from build123d import *

# Parameters (mm, degrees)
SKETCH1_W            = 34.3
SKETCH1_H            = 23.85
SKETCH1_W_2          = 24.3
SKETCH1_H_2          = 13.85
BOSS_EXTRUDE1_DEPTH  = 2
SKETCH4_W            = 8
SKETCH4_H            = 5
BOSS_EXTRUDE2_DEPTH  = 2
M2_CLEARANCE_HOLE1_D = 2.4
FILLET1_R            = 1
CUT_EXTRUDE1_DEPTH   = 3
FILLET2_R            = 0.25


with BuildPart() as part:
    # Sketch1 → Boss-Extrude1 (new body)
    with BuildSketch(Plane(origin=(0, 0, 0), x_dir=(1, 0, 0), z_dir=(0, 1, 0))):
        Rectangle(SKETCH1_W, SKETCH1_H)
        Rectangle(SKETCH1_W_2, SKETCH1_H_2, mode=Mode.SUBTRACT)
    extrude(amount=BOSS_EXTRUDE1_DEPTH)

    # Sketch4 → Boss-Extrude2 (add)
    with BuildSketch(Plane(origin=(0, 2, 0), x_dir=(1, 0, 0), z_dir=(0, 1, 0))):
        with Locations((-21.15, 0)):
            Rectangle(SKETCH4_W, SKETCH4_H)
        with Locations((21.15, 0)):
            Rectangle(SKETCH4_W, SKETCH4_H)
    extrude(amount=-BOSS_EXTRUDE2_DEPTH)

    # M2 Clearance Hole1 (through all)
    with Locations(Plane(origin=(0, 2, 0), x_dir=(1, 0, 0), z_dir=(0, 1, 0))):
        with Locations((-13.975, 0), (13.975, 0), (-21.475, 0), (21.475, 0)):
            Hole(M2_CLEARANCE_HOLE1_D / 2)

    # Fillet1
    fillet1_edges = [part.edges().sort_by_distance(p)[0] for p in [
        (-17.15, 1, -2.5),
        (-17.15, 1, 2.5),
        (-25.15, 1, 2.5),
        (-25.15, 1, -2.5),
        (17.15, 1, 2.5),
        (17.15, 1, -2.5),
        (25.15, 1, -2.5),
        (25.15, 1, 2.5),
        (-17.15, 1, -11.925),
        (17.15, 1, -11.925),
        (17.15, 1, 11.925),
        (-17.15, 1, 11.925),
    ]]
    fillet(fillet1_edges, radius=FILLET1_R)

    # Sketch5 → Cut-Extrude1 (cut, through all)
    with BuildSketch(Plane(origin=(0, 2, 0), x_dir=(1, 0, 0), z_dir=(0, 1, 0))):
        with BuildLine():
            Line((-12.15, 1.2), (-15.15, 1.2))
            ThreePointArc((-15.15, 1.2), (-16.35, 0), (-15.15, -1.2))
            Line((-15.15, -1.2), (-12.15, -1.2))
            Line((-12.15, -1.2), (-12.15, 1.2))
        make_face()
        with BuildLine():
            Line((12.15, 1.2), (15.15, 1.2))
            ThreePointArc((15.15, 1.2), (16.35, 0), (15.15, -1.2))
            Line((15.15, -1.2), (12.15, -1.2))
            Line((12.15, -1.2), (12.15, 1.2))
        make_face()
    extrude(amount=-CUT_EXTRUDE1_DEPTH, mode=Mode.SUBTRACT)

    # Fillet2
    fillet2_edges = [part.edges().sort_by_distance(p)[0] for p in [
        (-12.15, 1, 1.2),
        (-12.15, 1, -1.2),
        (12.15, 1, -1.2),
        (12.15, 1, 1.2),
    ]]
    fillet(fillet2_edges, radius=FILLET2_R)


solid = part.part
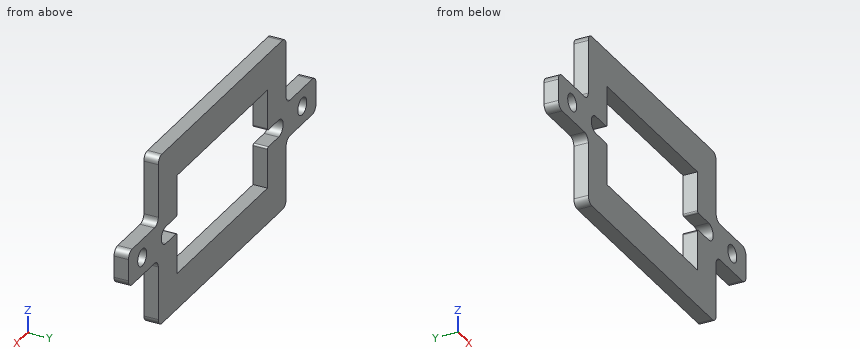
For this review, take the finished solid that the model builds, in its own axes (mm). Give positions to 0.01 mm unless a question says otherwise; leave off trailing zeros. Loops run counter-clockwise (first coordinate to the right, second up) from the corner with the lowest first, then second, coordinate; pieces in that order, holes last. Notation, with made-up numbers: M -7,86.5 L 4,86.5 A11 ccw 4,91.5 Z; hole C 87.5,-2 d4. An arc over 180 degrees is marked long. Answer as a JSON object with one key per item and string values. Group by question number.
Q1. Add section C-C on z = -5.75. Give the boundary of the cut face in (x, y).
Q2. Insertion check: P1, Ø1, axis at y = 1, z = 5.5, coming from the -X side. The pin has a flat end and moves straight along its axis. Give the tip position at first contact, or say it passes through.
Q3. Add section B-B on x = -1. Give the boundary of the cut face in (y, z) (3 decimals).
Q4. Add section D-D on y = 0.9. Give the number of separate pieces and of enclosed holes in the cut face, and give its area (3 significant figures).
Q5. For probe 1 along Z at (x, y) = (-2, 1.5) (3 decimals); probe 2 along X at (y, z) = (1.1, 6); probe 3 along Z at (x, y) = (13, 1.3) (3 decimals), list the stretches that pass through material, from the lowest coordinate up. Write a range as [from, to].
Q6. Add section A-A on z = 0. Give the boundary of the cut face in (x, y) (3 decimals), and give its area (3 significant figures).
Checked values:
{
 "1": {"outline": "M -17.15,0 L -12.15,0 L -12.15,2 L -17.15,2 Z; M 12.15,0 L 17.15,0 L 17.15,2 L 12.15,2 Z"},
 "2": {"P1": "x = -17.15"},
 "3": {"outline": "M 0,-11.925 L 2,-11.925 L 2,-6.925 L 0,-6.925 Z; M 0,6.925 L 2,6.925 L 2,11.925 L 0,11.925 Z"},
 "4": {"separate pieces": "1", "enclosed holes": "3", "area": "533 mm²"},
 "5": {"probe 1": "[-11.925, -6.925], [6.925, 11.925]", "probe 2": "[-17.15, -12.15], [12.15, 17.15]", "probe 3": "[-11.925, -1.2], [1.2, 11.925]"},
 "6": {"outline": "M -25.15,0 L -22.675,0 L -22.675,2 L -25.15,2 Z; M -20.275,0 L -16.35,0 L -16.35,2 L -20.275,2 Z; M 16.35,0 L 20.275,0 L 20.275,2 L 16.35,2 Z; M 22.675,0 L 25.15,0 L 25.15,2 L 22.675,2 Z", "area": "25.6 mm²"}
}
